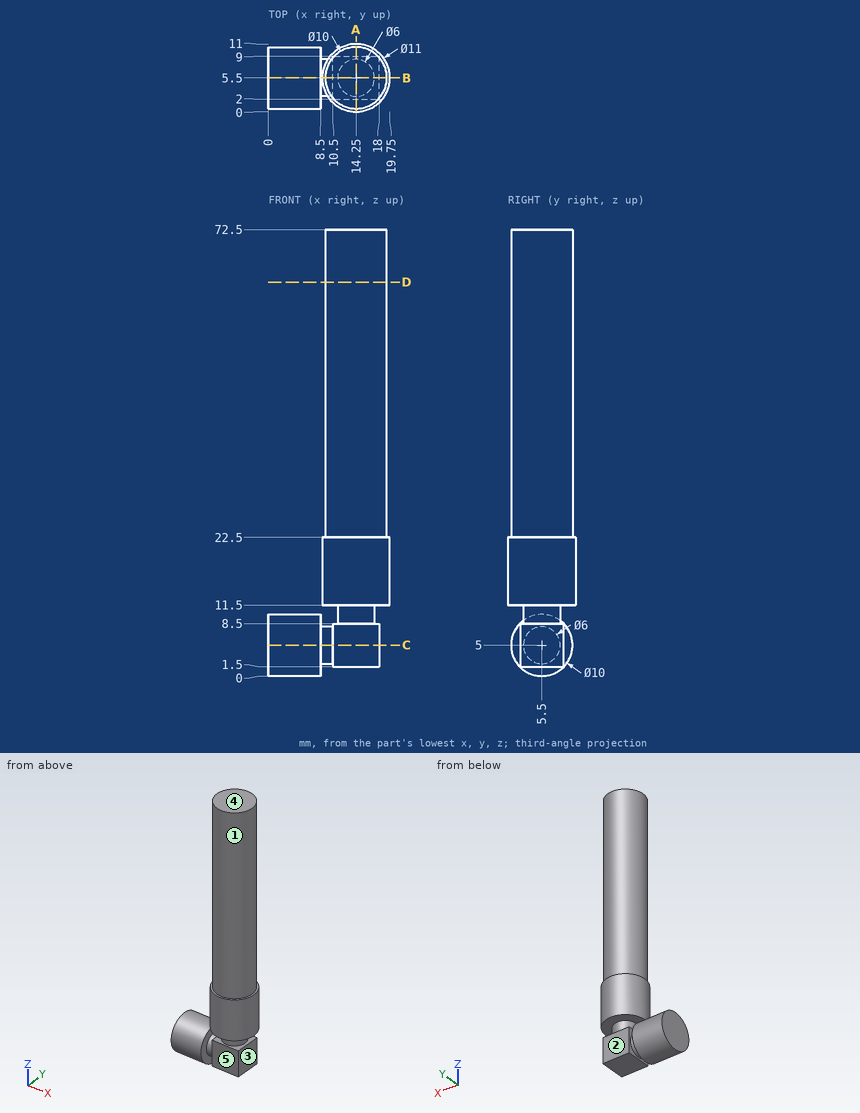
Study the drawing (mm; zero at the part's minimum x, y, z) and answer. A direction names the side the tool comes from. Give positions to 0.01 mm unless a question says otherwise; leave off trailing zeros. Write each loop counter-clockwise with the first axis right and the second up, starting at its lowest first coordinate (ties: lowest second). Pieces come first, ordered by that corner, then holes. Notation, with made-up numbers: (20.25, -27) -> (46.25, -27) arc R14 cw to (46.25, -4) -> close; hole circle Ø6 at (-17, 22). An arc over 180 degrees is marked (long way). Write item = value, one per line.
Q1. Consider line 1 along Y through (x, z) = (10, 13); line 2 along Z through (x, y) = (14.25, 9.75); line 3 along Y through (x, z) = (14, 62). Determine where each line is inside the solid, lowest interval first.
Computed values:
line_1 = 2.01 to 8.99
line_2 = 11.5 to 72.5
line_3 = 0.51 to 10.49
Q2. Section D-D on z = 64 is taken. Determine the outline of the cut face in (x, y), and give its area (3 significant figures).
Computed values:
outline = circle Ø10 at (14.25, 5.5)
area = 78.5 mm^2
Q3. Flat-ended cylindrical pins translate along their axes: pin 1 Ø5.5 at (x, y) = (16, 4.5) entering from -Z; pin 2 Ø3 at (y, z) = (2, 48.5) entering from -X; pin 3 Ø4 at (y, z) = (4, 65) entering from +X; pin 4 Ø4 at (x, z) = (2, 13.5) entering from +Y. Find the tip coordinate at first contact, or state that the pin passes through.
Computed values:
pin_1 = 1.5
pin_2 = 9.67
pin_3 = 19.25
pin_4 = through
Q4. Section A-A on x = 14.25 is taken. Determine the outline of the cut face in (y, z), and give its area (3 significant figures).
Computed values:
outline = (0, 11.5) -> (2.5, 11.5) -> (2.5, 8.5) -> (2, 8.5) -> (2, 1.5) -> (9, 1.5) -> (9, 8.5) -> (8.5, 8.5) -> (8.5, 11.5) -> (11, 11.5) -> (11, 22.5) -> (10.5, 22.5) -> (10.5, 72.5) -> (0.5, 72.5) -> (0.5, 22.5) -> (0, 22.5) -> close
area = 688 mm^2
Q5. Section B-B on y = 5.5 is taken. Determine the outline of the cut face in (x, z).
Computed values:
outline = (0, 0) -> (8.5, 0) -> (8.5, 2) -> (10.5, 2) -> (10.5, 1.5) -> (18, 1.5) -> (18, 8.5) -> (17.25, 8.5) -> (17.25, 11.5) -> (19.75, 11.5) -> (19.75, 22.5) -> (19.25, 22.5) -> (19.25, 72.5) -> (9.25, 72.5) -> (9.25, 22.5) -> (8.75, 22.5) -> (8.75, 11.5) -> (11.25, 11.5) -> (11.25, 8.5) -> (10.5, 8.5) -> (10.5, 8) -> (8.5, 8) -> (8.5, 10) -> (0, 10) -> close
Q6. A tool of negligible diameter and unlimited length cuts with its end or side. For the marked faces 1, 2, 3, 4 and 5, from which of +Z, -Z, +X, -X, +Y, -Y can it reach the whole face along a straight path? Write none if from no direction.
Computed values:
face_1 = +Z
face_2 = -Z, +X, +Y
face_3 = -Z, +X, +Y, -Y
face_4 = +Z, +X, -X, +Y, -Y
face_5 = -Z, +X, -Y
Q7. Section C-C on z = 5 is taken. Determine the outline of the cut face in (x, y), and give its area (4 significant figures).
Computed values:
outline = (0, 0.5) -> (8.5, 0.5) -> (8.5, 2.5) -> (10.5, 2.5) -> (10.5, 2) -> (18, 2) -> (18, 9) -> (10.5, 9) -> (10.5, 8.5) -> (8.5, 8.5) -> (8.5, 10.5) -> (0, 10.5) -> close
area = 149.5 mm^2
